Verification items for the finished model (mm, model axes). Face numbers are marked on the shaded views. A direction names the side the tool comes from. Coordinates: 2 decimals unless noted, no trailing zeros. Write each loop counter-clockwise with the first axis right and the second up, starting at its lowest first coordinate (ties: lowest second). Pieces come first, ordered by that corner, then holes. Notation, with made-up numbers: (88, 18.5) -> (133, 18.5) arc R14 cw to (133, 42.5) -> close; hole circle Ø2 at (37.25, 36). An arc over 180 degrees is marked (long way). Write item = value, one per line. Start each with the question number.
(1) Section check A-A (z = 0). Record the cut outline in (x, y) (1 decimal).
(2) Gauge pin test, flat end, axial feed: pin 1 Ø1.5 at (x, z) = (-11.5, 1.5) entering from +Y. Record the tip position at first contact, or that the pin passes through.
(3) Section check C-C (x = 16.5). Record the cut outline in (y, z), plus the area to 3 significant figures.
(4) Set-up check for the marked faces 1 and 2: record each of +Z, -Z, +X, -X, +Y, -Y from which the full face is reachable in a straight line by a thin tool's end or side.
(5) Material ranges on probe 1 along Y at (x, z) = (28.75, 0) (3 decimals); probe 2 along X at (y, z) = (0.45, 1.65); probe 3 along X at (y, z) = (-0.05, 0.6), recorded low to high. Write a range as [from, to].
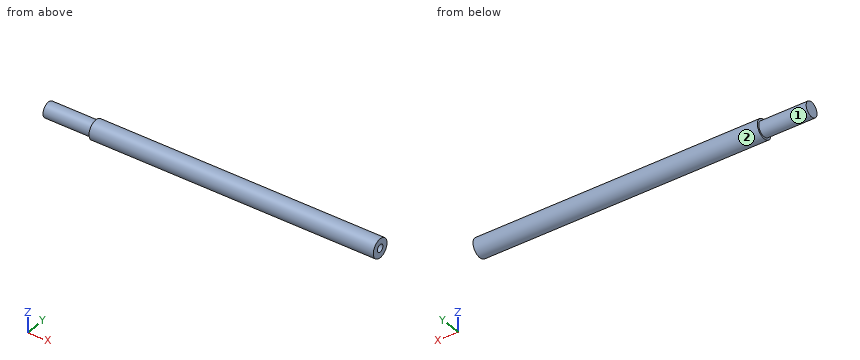
```python
from build123d import *

# Parameters (mm, degrees)
SKETCH1_R           = 2
BOSS_EXTRUDE1_DEPTH = 30
SKETCH2_R           = 0.795
CUT_EXTRUDE1_DEPTH  = 7
SKETCH3_R           = 1.5875
BOSS_EXTRUDE2_DEPTH = 10


with BuildPart() as part:
    # Sketch1 → Boss-Extrude1 (new, symmetric)
    with BuildSketch(Plane(origin=(0, 0, 0), x_dir=(0, 0, -1), z_dir=(1, 0, 0))):
        Circle(SKETCH1_R)
    extrude(amount=BOSS_EXTRUDE1_DEPTH, both=True)

    # Sketch2 → Cut-Extrude1 (cut)
    with BuildSketch(Plane(origin=(30, 0, 0), x_dir=(0, 0, -1), z_dir=(1, 0, 0))):
        Circle(SKETCH2_R)
    extrude(amount=-CUT_EXTRUDE1_DEPTH, mode=Mode.SUBTRACT)

    # Sketch3 → Boss-Extrude2 (add)
    with BuildSketch(Plane.ZY.offset(30)):
        with Locations(Location((0, 0, 0), (0, 0, 180))):
            Circle(SKETCH3_R)
    extrude(amount=BOSS_EXTRUDE2_DEPTH)


solid = part.part
```
Response:
q1.outline = (-40, -1.6) -> (-30, -1.6) -> (-30, -2) -> (30, -2) -> (30, -0.8) -> (23, -0.8) -> (23, 0.8) -> (30, 0.8) -> (30, 2) -> (-30, 2) -> (-30, 1.6) -> (-40, 1.6) -> close
q2.pin_1 = 1.85
q3.outline = circle Ø4 at (0, 0)
q3.area = 12.6 mm2
q4.face_1 = -X
q4.face_2 = +X, -X
q5.probe_1 = [-2, -0.795], [0.795, 2]
q5.probe_2 = [-30, 30]
q5.probe_3 = [-40, 23]
